For this review, take the finished solid that the model builds, in its own axes (mm). A direction names the side the tool comes from. Coordinates: 2 decimals unless noted, no trailing zeros. Loops run counter-clockwise (first coordinate to the right, second up) from the corner with the lowest first, then second, coordinate; pieces in that order, holes last. Notation, with made-up numbers: (73.5, 58.5) -> (110.5, 58.5) arc R20 ccw to (110.5, 75.5) -> close; hole circle Ø7 at (0.5, 43). An arc over 180 degrees is marked (long way). Answer in a Markdown table with one row per item.
from build123d import *

# Parameters (mm, degrees)
BOSS_EXTRUDE1_DEPTH = 6.35
BOSS_EXTRUDE2_DEPTH = 8.7122
CUT_EXTRUDE1_START  = 2.54
SKETCH3_W           = 71.12
SKETCH3_H           = 57.15
CUT_EXTRUDE1_DEPTH  = 3.556
HOLE1_D             = 7.62
CUT_EXTRUDE2_DEPTH  = 10.6172
SKETCH8_W           = 22.86
SKETCH8_H           = 22.86
SKETCH8_W_2         = 17.78
SKETCH8_H_2         = 17.78
BOSS_EXTRUDE3_DEPTH = 10.6172
FILLET1_R           = 0.254
FILLET2_R           = 6.604
FILLET3_R           = 9.144
CHAMFER1_SIZE       = 1.016
BOSS_EXTRUDE4_DEPTH = 6.35


with BuildPart() as part:
    # Sketch1 → Boss-Extrude1 (new body)
    with BuildSketch(Plane(origin=(0, 0, 0), x_dir=(1, 0, 0), z_dir=(0, 1, 0))):
        with BuildLine():
            Line((-35.56, 21.431101635), (-35.56, -21.431101635))
            ThreePointArc((-35.56, -21.431101635), (0, -28.575), (35.56, -21.431101635))
            Line((35.56, -21.431101635), (35.56, 21.431101635))
            ThreePointArc((35.56, 21.431101635), (0, 28.575), (-35.56, 21.431101635))
        make_face()
    extrude(amount=-BOSS_EXTRUDE1_DEPTH)

    # Sketch2 → Boss-Extrude2 (add)
    with BuildSketch(Plane.XZ.offset(6.35)):
        with BuildLine():
            Line((30.7086, -18.139073262), (30.7086, 18.139073262))
            ThreePointArc((30.7086, 18.139073262), (0, 23.7236), (-30.7086, 18.139073262))
            Line((-30.7086, 18.139073262), (-30.7086, -18.139073262))
            ThreePointArc((-30.7086, -18.139073262), (0, -23.7236), (30.7086, -18.139073262))
        make_face()
    extrude(amount=BOSS_EXTRUDE2_DEPTH)

    # Sketch3 → Cut-Extrude1 (cut)
    with BuildSketch(Plane.XZ.offset(6.35).offset(CUT_EXTRUDE1_START)):
        Rectangle(SKETCH3_W, SKETCH3_H)
        with BuildLine():
            Line((28.9306, -16.898824264), (28.9306, 16.898824264))
            ThreePointArc((28.9306, 16.898824264), (0, 21.9456), (-28.9306, 16.898824264))
            Line((-28.9306, 16.898824264), (-28.9306, -16.898824264))
            ThreePointArc((-28.9306, -16.898824264), (0, -21.9456), (28.9306, -16.898824264))
        make_face(mode=Mode.SUBTRACT)
    extrude(amount=CUT_EXTRUDE1_DEPTH, mode=Mode.SUBTRACT)

    # Hole1 (through all)
    with Locations(Plane(origin=(0, -15.0622, 0), x_dir=(-1, 0, 0), z_dir=(0, -1, 0))):
        with Locations((0, 0)):
            Hole(HOLE1_D / 2)

    # Sketch7 → Cut-Extrude2 (cut)
    with BuildSketch(Plane.XZ.offset(15.0622)):
        with BuildLine():
            Line((25.6286, -14.54323086), (25.6286, 14.54323086))
            ThreePointArc((25.6286, 14.54323086), (0, 18.6436), (-25.6286, 14.54323086))
            Line((-25.6286, 14.54323086), (-25.6286, -14.54323086))
            ThreePointArc((-25.6286, -14.54323086), (0, -18.6436), (25.6286, -14.54323086))
        make_face()
    extrude(amount=-CUT_EXTRUDE2_DEPTH, mode=Mode.SUBTRACT)

    # Sketch8 → Boss-Extrude3 (add)
    with BuildSketch(Plane.XZ.offset(4.445)):
        Rectangle(SKETCH8_W, SKETCH8_H)
        Rectangle(SKETCH8_W_2, SKETCH8_H_2, mode=Mode.SUBTRACT)
    extrude(amount=BOSS_EXTRUDE3_DEPTH)

    # Fillet1
    fillet1_edges = [part.edges().sort_by_distance(p)[0] for p in [
        (0, -8.89, -21.9456),
        (28.9306, -8.89, 0),
        (0, -8.89, 21.9456),
        (-28.9306, -8.89, 0),
        (0, -12.446, -21.9456),
        (28.9306, -12.446, 0),
        (0, -12.446, 21.9456),
        (-28.9306, -12.446, 0),
    ]]
    fillet(fillet1_edges, radius=FILLET1_R)

    # Fillet2
    fillet2_edges = [part.edges().sort_by_distance(p)[0] for p in [
        (8.89, -9.7536, -8.89),
        (-8.89, -9.7536, -8.89),
        (-8.89, -9.7536, 8.89),
        (8.89, -9.7536, 8.89),
    ]]
    fillet(fillet2_edges, radius=FILLET2_R)

    # Fillet3
    fillet3_edges = [part.edges().sort_by_distance(p)[0] for p in [
        (-11.43, -9.7536, -11.43),
        (-11.43, -9.7536, 11.43),
        (11.43, -9.7536, 11.43),
        (11.43, -9.7536, -11.43),
    ]]
    fillet(fillet3_edges, radius=FILLET3_R)

    # Chamfer1
    chamfer1_edges = [part.edges().sort_by_distance(p)[0] for p in [
        (-8.89, -15.0622, 0),
        (0, -15.0622, -8.89),
        (8.89, -15.0622, 0),
        (0, -15.0622, 8.89),
        (-6.955733183, -15.0622, -6.955733183),
        (6.955733183, -15.0622, -6.955733183),
        (-6.955733183, -15.0622, 6.955733183),
        (6.955733183, -15.0622, 6.955733183),
        (-11.43, -15.0622, 0),
        (0, -15.0622, 11.43),
        (0, -15.0622, -11.43),
        (11.43, -15.0622, 0),
        (8.751784407, -15.0622, -8.751784407),
        (-8.751784407, -15.0622, -8.751784407),
        (8.751784407, -15.0622, 8.751784407),
        (-8.751784407, -15.0622, 8.751784407),
        (0, -15.0622, -18.6436),
        (25.6286, -15.0622, 0),
        (0, -15.0622, 18.6436),
        (-25.6286, -15.0622, 0),
    ]]
    chamfer(chamfer1_edges, length=CHAMFER1_SIZE)

    # Sketch9 → Boss-Extrude4 (add)
    with BuildSketch(Plane(origin=(0, 0, 0), x_dir=(1, 0, 0), z_dir=(0, 1, 0))):
        with BuildLine():
            Line((-3.175, 42.142831106), (3.175, 42.142831106))
            ThreePointArc((3.175, 42.142831106), (6.767102448, 40.654933554), (8.255, 37.062831106))
            ThreePointArc((8.255, 37.062831106), (10.610545149, 30.557749671), (16.584937888, 27.069009381))
            ThreePointArc((16.584937888, 27.069009381), (0, 28.575), (-16.584937888, 27.069009381))
            ThreePointArc((-16.584937888, 27.069009381), (-10.610545149, 30.557749671), (-8.255, 37.062831106))
            ThreePointArc((-8.255, 37.062831106), (-6.767102448, 40.654933554), (-3.175, 42.142831106))
        make_face()
    extrude(amount=-BOSS_EXTRUDE4_DEPTH)


solid = part.part
Item 1: Take a section at B-B, the plane z = -35. State the section outline as (x, y) points, and give its area (3 significant figures).
Worked answers:
| item | result |
|---|---|
| outline | (-8.47, -6.35) -> (8.47, -6.35) -> (8.47, 0) -> (-8.47, 0) -> close |
| area | 108 mm² |
Item 2: Insertion check: pin 1 (1.3 mm diameter, centred on y = -7.5, z = 3.5, fed in from -X); pin 2 (3 mm diameter, centred on y = -10, z = 4, fed in from +X); pin 3 (1 mm diameter, centred on x = -21.5, y = -10.5, fed in from +Z). Each pin has a flat end and moves straight along its axis. Give the tip position at first contact, or say it passes through.
Worked answers:
| item | result |
|---|---|
| pin 1 | x = -30.71 |
| pin 2 | x = 30.71 |
| pin 3 | z = 19.32 |
Item 3: Take a section at A-A, the plane y = -3.25. State the section outline as (x, z) points (3 decimals), and give its area (3 significant figures).
Worked answers:
| item | result |
|---|---|
| outline | (-35.56, -21.431) arc R92.075 ccw to (-16.585, -27.069) arc R10.16 cw to (-8.255, -37.063) arc R5.08 ccw to (-3.175, -42.143) -> (3.175, -42.143) arc R5.08 ccw to (8.255, -37.063) arc R10.16 cw to (16.585, -27.069) arc R92.075 ccw to (35.56, -21.431) -> (35.56, 21.431) arc R92.075 ccw to (-35.56, 21.431) -> close; hole circle Ø7.62 at (0, 0) |
| area | 3,930 mm² |
Item 4: The part is to be moulded in two halves that separate along Z. For faces 1 (the cylindrical face through (-0.439, -13.736, -23.722)), 2 (the flat face through (11.43, -9, 0)), 3 (the flat face through (30.709, -14, 0)), say which applies: +Z half, -Z half, draft (parallel to the pull), parting line (faces both ways), or undercut.
Worked answers:
| item | result |
|---|---|
| face 1 | -Z half |
| face 2 | undercut |
| face 3 | draft |
Item 5: For faces 4 (the cylindrical face through (0.413, -10.647, 21.945)), 5 (the conical face through (7.12, -14.21, -7.02)), 6 (the flat face through (0, -15.062, 10.1)), list the 3-axis set-ups (+Z, -Z, +X, -X, +Y, -Y) from which the entire face can be reached by the end or side of a thin tool; tool diameter is ignored.
Worked answers:
| item | result |
|---|---|
| face 4 | +Z |
| face 5 | -Y |
| face 6 | +Z, -Z, +X, -X, -Y |
Item 6: For L1, parallel to Y at x = -30.5, z = -7; L2, parallel to X at y = -11.25, z = -12; L3, parallel to Z at x = 0, y = -1.2 (3 decimals), list the stretches that pass through material, from the lowest coordinate up.
Worked answers:
| item | result |
|---|---|
| L1 | -15.06 to -12.45, -8.89 to 0 |
| L2 | -28.93 to -25.63, 25.63 to 28.93 |
| L3 | -42.143 to -3.81, 3.81 to 28.575 |
